Could you check a few things on this model? Use its own coordinates, in mm. A direction names the side the tool comes from. Coordinates: 2 decimals unless noted, no trailing zeros. Order: outer loops, then holes, each group sorted by start corner. A loop starts at its lowest first (then second) coordinate and runs counter-clockwise, first axis right, second up. Notation, with made-up numbers: (-18.75, -27.75) - (39.25, -27.75) arc R18 cw to (39.25, -4.75) - close; hole circle Ø5 at (-34.5, 1). An arc over 180 degrees is marked (long way). One line per item, written item: value.
Autodesk Inventor part; units mm, degrees
ref_plane "YZ Plane" through (0, 0, 0) normal (1, 0, 0) x (0, 1, 0)
ref_plane "XZ Plane" through (0, 0, 0) normal (0, 1, 0) x (-1, 0, 0)
ref_plane "XY Plane" through (0, 0, 0) normal (0, 0, 1) x (1, 0, 0)
sketch "草圖1" plane through (0, 0, 0) normal (0, 0, 1) x (1, 0, 0)
  line L0 (0, 7.9) -> (5, 7.9)
  line L1 (5, 7.9) -> (5, 1.6)
  line L2 (5, 1.6) -> (15, 1.6)
  line L3 (15, 1.6) -> (15, 0)
  line L4 (15, 0) -> (0, 0)
  line L5 (0, 7.9) -> (0, 0)
  point P0 (0, 0)
  dimension "d1" = 1.6
  dimension "d2" = 10
  dimension "d3" = 30
  dimension "d4" = 6.3
revolve "迴轉1" add sketch "草圖1" angle 360 about axis through (0, 7.9, 0) along (0, -1, 0)
sketch "草圖2" plane through (0, 0, 0) normal (0, 1, 0) x (-1, 0, 0)
  line L0 (12.5, -5.5) -> (-12.5, -5.5)
  line L1 (-12.5, -5.5) -> (-12.5, 5.5)
  line L2 (-12.5, 5.5) -> (12.5, 5.5)
  line L3 (12.5, 5.5) -> (12.5, -5.5)
  circle A0 centre (10, 0) radius 1.6
  circle A1 centre (-10, 0) radius 1.6
  line L4 (10, 0) -> (-10, 0) construction
  point P0 (0, 0)
  point P1 (0, -5.5)
  point P2 (-12.5, 0)
  point P3 (0, 0)
  dimension "d6" = 11
  dimension "d7" = 25
  dimension "d8" = 3.2
  dimension "d9" = 20
extrude "擠出1" cut sketch "草圖2" along normal through all keep common part
properties part number "磁鐵b" material "SS41"
Item 1: I want a section at A-A on z = 0. Please give me the cut outline in (x, y), then the cut area to 3 significant figures.
Conclusion:
outline: (-12.5, 0) - (-11.6, 0) - (-11.6, 1.6) - (-12.5, 1.6) - close; (-8.4, 0) - (8.4, 0) - (8.4, 1.6) - (5, 1.6) - (5, 7.9) - (-5, 7.9) - (-5, 1.6) - (-8.4, 1.6) - close; (11.6, 0) - (12.5, 0) - (12.5, 1.6) - (11.6, 1.6) - close
area: 92.8 mm²
Item 2: If I drill on probe 1 along X at (y, z) = (0.7, 0); probe 2 along Z at (x, y) = (10, 1); probe 3 along Y at (x, z) = (-7.5, -2), over which ranges is the centre line in solid material (lowest first)?
Conclusion:
probe 1: -12.5 to -11.6, -8.4 to 8.4, 11.6 to 12.5
probe 2: -5.5 to -1.6, 1.6 to 5.5
probe 3: 0 to 1.6
Item 3: Thinking about a two-plate mould opening in X: for faces 3 (the face through (-12.5, 1, 0)), 4 (the face through (0, 7.9, 0)), 5 (the face through (11.6, 0.79, -0.07)), which applies, pulls with the +X half, pulls with the -X half, needs draft (parallel to the pull), parting line crosses it, or undercut?
Conclusion:
face 3: pulls with the -X half
face 4: needs draft
face 5: undercut
Item 4: I want a section at B-B on x = 10. Please give me the cut outline in (y, z).
Conclusion:
outline: (0, -5.5) - (1.6, -5.5) - (1.6, -1.6) - (0, -1.6) - close; (0, 1.6) - (1.6, 1.6) - (1.6, 5.5) - (0, 5.5) - close
Item 5: I want a section at D-D on z = -4.25. Please give me the cut outline in (x, y).
Conclusion:
outline: (-12.5, 0) - (12.5, 0) - (12.5, 1.6) - (2.63, 1.6) - (2.63, 7.9) - (-2.63, 7.9) - (-2.63, 1.6) - (-12.5, 1.6) - close
Item 6: I want a section at C-C on x = 0. Please give me the cut outline in (y, z), then the cut area to 3 significant figures.
Conclusion:
outline: (0, -5.5) - (1.6, -5.5) - (1.6, -5) - (7.9, -5) - (7.9, 5) - (1.6, 5) - (1.6, 5.5) - (0, 5.5) - close
area: 80.6 mm²
Item 7: For faces 1 (the face through (0, 0, 0)), 2 (the face through (-1.08, 4.71, -4.88)), which set-ups out of +Z, -Z, +X, -X, +Y, -Y let a thin tool reach every point of the face, with its end or its side?
Conclusion:
face 1: +Z, -Z, +X, -X, -Y
face 2: +Y
Item 8: I'm going to push flat-ended pins straight in: pin 1 Ø2 at (x, y) = (1, 5) entering from -Z; pin 2 Ø6 at (x, z) = (9.5, -3.5) entering from +Y; pin 3 Ø2.5 at (x, z) = (-10, 0) entering from +Y; pin 4 Ø2 at (y, z) = (6, -2) entering from +X. Where does each tip first touch, or does it pass through?
Conclusion:
pin 1: z = -5
pin 2: y = 1.6
pin 3: through
pin 4: x = 4.9
